Geometry: final body of the model. Coordinates: model frame, mm. Face numbers are marked on the shaded views. A direction names the side the tool comes from. Give positions to 0.01 mm unless a question says otherwise; leave off trailing zeros. Order: outer loops, then holes, each group sorted by start corner. A loop starts at its lowest first (then second) coordinate and runs counter-clockwise, first axis right, second up. Notation, with made-up numbers: M -39.75,-29.5 L -30.75,-29.5 A13 ccw -30.75,-9.5 Z; hole C 70,57 d5. An arc over 180 degrees is marked long. Use CSV: the item, a comma, the result in double quotes.
```python
from build123d import *

# Parameters (mm, degrees)
SKETCH1_W                  = 54.5
SKETCH1_H                  = 111
BOSS_EXTRUDE1_DEPTH        = 4.5
SKETCH2_W                  = 13.5
SKETCH2_H                  = 111
BOSS_EXTRUDE2_DEPTH        = 12.5
M4X0_7_TAPPED_HOLE1_D      = 3.3
SKETCH6_W                  = 4
SKETCH6_H                  = 12.5
BOSS_EXTRUDE3_DEPTH        = 37
SKETCH7_W                  = 54.5
SKETCH7_H                  = 3
BOSS_EXTRUDE5_DEPTH        = 39
SKETCH8_R                  = 7
CUT_EXTRUDE1_DEPTH         = 3
M2_CLEARANCE_HOLE1_D       = 2.4
F_8_0_199_DIAMETER_HOLE1_D = 5.0546
SKETCH12_R                 = 5.5
CUT_EXTRUDE3_DEPTH         = 3
SKETCH13_W                 = 27.5
SKETCH13_H                 = 9.513667368
CUT_EXTRUDE4_DEPTH         = 5


with BuildPart() as part:
    # Sketch1 → Boss-Extrude1 (new body)
    with BuildSketch(Plane(origin=(0, 0, 0), x_dir=(1, 0, 0), z_dir=(0, 1, 0))):
        with Locations((-13.399543841, 44.129312584)):
            Rectangle(SKETCH1_W, SKETCH1_H)
    extrude(amount=BOSS_EXTRUDE1_DEPTH)

    # Sketch2 → Boss-Extrude2 (add)
    with BuildSketch(Plane(origin=(0, 4.5, 0), x_dir=(1, 0, 0), z_dir=(0, 1, 0))):
        with Locations((7.100456159, 44.129312584)):
            Rectangle(SKETCH2_W, SKETCH2_H)
        with Locations((-33.899543841, 44.129312584)):
            Rectangle(SKETCH2_W, SKETCH2_H)
    extrude(amount=BOSS_EXTRUDE2_DEPTH)

    # M4x0.7 Tapped Hole1 (through all)
    with Locations(Plane(origin=(-31.949543841, 17, -9.129312584), x_dir=(0, 0, 1), z_dir=(0, 1, 0))):
        with Locations((0, 0), (-25, 0), (-50, 0), (-75, 0), (0, 37.1), (-25, 37.1), (-50, 37.1), (-75, 37.1)):
            Hole(M4X0_7_TAPPED_HOLE1_D / 2)

    # Sketch6 → Boss-Extrude3 (add)
    with BuildSketch(Plane(origin=(-27.149543841, 0, 0), x_dir=(0, 0, -1), z_dir=(1, 0, 0))):
        with Locations((-9.370687416, 10.75)):
            Rectangle(SKETCH6_W, SKETCH6_H)
    extrude(amount=BOSS_EXTRUDE3_DEPTH)

    # Sketch7 → Boss-Extrude5 (add)
    with BuildSketch(Plane.XY.offset(11.370687416)):
        with Locations((-13.399543841, 15.5)):
            Rectangle(SKETCH7_W, SKETCH7_H)
    extrude(amount=BOSS_EXTRUDE5_DEPTH)

    # Sketch8 → Cut-Extrude1 (cut)
    with BuildSketch(Plane(origin=(0, 17, 0), x_dir=(1, 0, 0), z_dir=(0, 1, 0))):
        with Locations((-13.399543841, -30.870687416)):
            Circle(SKETCH8_R)
    extrude(amount=-CUT_EXTRUDE1_DEPTH, mode=Mode.SUBTRACT)

    # M2 Clearance Hole1 (through all)
    with Locations(Plane(origin=(-21.371437118, 17, 30.847906254), x_dir=(0, 0, 1), z_dir=(0, 1, 0))):
        with Locations((0, 0), (-7.977218838, 7.971893277), (8.022781162, 7.971893277), (-0.002806072, 15.940961576)):
            Hole(M2_CLEARANCE_HOLE1_D / 2)

    # #8 (0.199) Diameter Hole1 (through all)
    with Locations(Plane(origin=(-13.399543841, 4.5, 2.370687416), x_dir=(0, 0, 1), z_dir=(0, 1, 0))):
        with Locations((0, 0), (-10, 0), (-35, 0), (-85, 0), (-95, 0)):
            Hole(F_8_0_199_DIAMETER_HOLE1_D / 2)

    # Sketch12 → Cut-Extrude3 (cut)
    with BuildSketch(Plane(origin=(0, 0, 0), x_dir=(-1, 0, 0), z_dir=(0, -1, 0))):
        with Locations((13.399543841, 92.629312584)):
            Circle(SKETCH12_R)
    extrude(amount=-CUT_EXTRUDE3_DEPTH, mode=Mode.SUBTRACT)

    # Sketch13 → Cut-Extrude4 (cut)
    with BuildSketch(Plane.XY.offset(11.370687416)):
        with Locations((-13.399543841, 9.243166316)):
            Rectangle(SKETCH13_W, SKETCH13_H)
    extrude(amount=-CUT_EXTRUDE4_DEPTH, mode=Mode.SUBTRACT)


solid = part.part
```
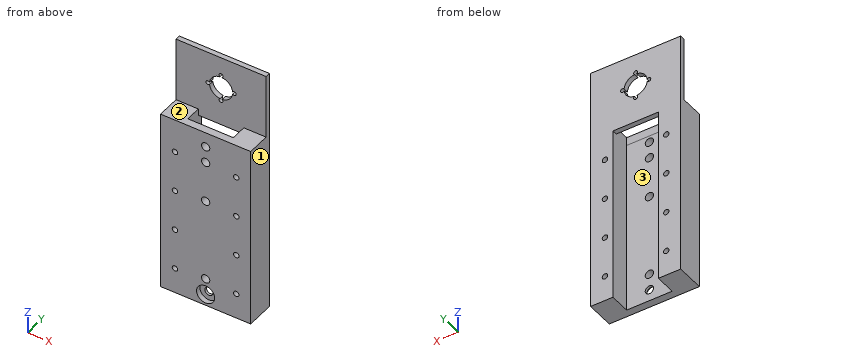
1. Section B-B, the plane y = 9.5. Give the number of separate pieces and of enclosed holes in the cut face, plus the area to 3 significant figures.
Answer:
separate pieces,"2"
enclosed holes,"8"
area,"2,930 mm2"
2. Section C-C, the plane z = -26.5. Return the cut outline in (x, y), plus the area to 3 significant figures.
Answer:
outline,"M -40.65,0 L 13.85,0 L 13.85,17 L 0.35,17 L 0.35,4.5 L -27.15,4.5 L -27.15,17 L -40.65,17 Z"
area,"583 mm2"
3. Section A-A, the plane z = 36.5. Return the cut outline in (x, y).
Answer:
outline,"M -40.65,14 L -17.56,14 L -17.56,17 L -40.65,17 Z; M -9.24,14 L 13.85,14 L 13.85,17 L -9.24,17 Z"
4. Line query: line 1 (X direction, y = 5.75, z = -31); line 2 (X direction, y = 10.75, z = -59.5); line 3 (X direction, y = 9.5, z = -58). Output: solid intervals per line, ascending.
Answer:
line 1,"-40.65 to -27.15, 0.35 to 13.85"
line 2,"-40.65 to -33.56, -30.34 to -27.15, 0.35 to 3.54, 6.76 to 13.85"
line 3,"-40.65 to -33.15, -30.75 to -27.15, 0.35 to 3.95, 6.35 to 13.85"
5. Reachability of the marked faces 1, 2 and 3 from +Z, -Z, +X, -X, +Y, -Y: full face, straight path, thin tool, end or side. Return the list, or none.
Answer:
face 1,"+Z, -Z, +X, +Y, -Y"
face 2,"+Z, +X, -X, -Y"
face 3,"+Z, -Z, +Y"
6. Pin query (flat end, axial travel): pin 1 Ø1 at (x, z) = (-9.5, -36) entering from +Y. Return the tip coordinate at first contact, or that it passes through.
Answer:
pin 1,"y = 4.5"
